Verification items for the finished model (mm, model axes). A direction names the side the tool comes from. Give positions to 0.01 mm unless a question says otherwise; leave off trailing zeros. Order: outer loops, then holes, each group sorted by start corner. A loop starts at its lowest first (then second) coordinate and runs counter-clockwise, first axis right, second up.
(1) Gauge pin test, flat ends, axial feed: pin 1 (1.2 mm diameter, centred on y = 44, z = 7.5, fed in from -X); pin 2 (4 mm diameter, centred on x = 20.17, y = 37.33, fed in from +Z); pin 3 (1.5 mm diameter, centred on x = 28, z = 3, fed in from -Y). Record the tip position at first contact, or that the pin passes through.
(2) Access from +Z, -Z, +X, -X, +Y, -Y to the whole of each face (thin tool, end or side, straight path). Record for faces 5 (the face through (21.836, 37.859, 6.084)), 6 (the face through (20.857, 39.996, 14.535)), 7 (the face through (10, 3, 7)).
(3) Sectioned sample at B-B on y = 20. Record the cut outline in (x, z).
(4) Mould release check, pull along X, two halves, no side actions. Record for faces 1 (the face through (42, 31, 8)), 2 (the face through (18, 32, 7)), 3 (the face through (33.794, 23.738, 14.535)), 4 (the face through (10, 60, 7)): pulls with the +X half, pulls with the -X half, needs draft (parallel to the pull), parting line crosses it, or undercut.
(5) Scan lines: L1, parallel to Y at x = 26, z = 9; L2, parallel to Z at x = 12, y = 17; L3, parallel to Y at x = 32, z = 14. Record each from-to range of solid material in increasing order.
(6) Sectioned sample at C-C on x = 26. Count the separate pieces of the cut face and the enclosed holes in it, plus the area to 3 significant figures.
(7) Sectioned sample at A-A on y = 31.5. Record the cut outline in (x, z), plus the area to 3 significant figures.
(8) Sectioned sample at D-D on y = 11.5. Record the cut outline in (x, z).
Autodesk Inventor part; units mm, degrees
ref_plane "Work Plane2" through (3, 0, 0) normal (-1, 0, 0) x (0, 0, 1)
ref_plane "YZ Plane" through (0, 0, 0) normal (1, 0, 0) x (0, 1, 0)
ref_plane "XZ Plane" through (0, 0, 0) normal (0, 1, 0) x (-1, 0, 0)
sketch "Sketch1" plane through (0, 0, 0) normal (0, 0, 1) x (1, 0, 0)
  line L0 (0, 0) -> (42, 0)
  line L1 (42, 0) -> (42, 63)
  line L2 (42, 63) -> (0, 63)
  line L3 (0, 63) -> (0, 0)
  dimension "d0" = 42
  dimension "d1" = 63
extrude "Extrusion1" add sketch "Sketch1" along normal blind 17
sketch "Sketch2" plane through (0, 0, 17) normal (0, 0, 1) x (1, 0, 0)
  line L0 (0, 63) -> (0, 0)
  line L1 (0, 31.5) -> (26, 31.5)
  circle A0 centre (26, 31.5) radius 5.25
  dimension "d4" = 26
  dimension "d5" = 10.5
extrude "Extrusion2" cut sketch "Sketch2" against normal blind 17
sketch "Sketch4" plane through (0, 0, 17) normal (0, 0, 1) x (1, 0, 0)
  circle A0 centre (26, 31.5) radius 5.25
  line L0 (26, 31.5) -> (26, 51.5)
  line L1 (26, 31.5) -> (26, 11.5)
  circle A1 centre (26, 51.5) radius 7.55
  circle A2 centre (26, 11.5) radius 7.55
  point P0 (0, 0)
  dimension "d14" = 20
  dimension "d15" = 20
  dimension "d16" = 15.1
  dimension "d17" = 15.1
extrude "Extrusion4" cut sketch "Sketch4" against normal blind 17 contours A2 | A1
sketch "Sketch5" plane through (0, 0, 17) normal (0, 0, 1) x (1, 0, 0)
  line L0 (0, 63) -> (0, 0)
  line L1 (0, 31.5) -> (10, 31.5)
  circle A0 centre (26, 31.5) radius 5.25
  line L2 (26, 31.5) -> (20.1664, 37.3336)
  line L3 (26, 31.5) -> (34.25, 31.5) construction
  line L4 (20.1664, 37.3336) -> (31.8336, 25.6664)
  circle A1 centre (31.8336, 25.6664) radius 1.75
  circle A2 centre (20.1664, 37.3336) radius 1.75
  dimension "d21" = 10
  dimension "d22" = 8.25
  dimension "d23" = 135
  dimension "d24" = 16.5
  dimension "d25" = 3.5
  dimension "d26" = 3.5
extrude "Extrusion5" cut sketch "Sketch5" against normal blind 17 contours A1 | A2
ref_plane "Work Plane1" through (0, 0, 7.5) normal (0, 0, 1) x (1, 0, 0)
sketch "Sketch8" plane through (0, 0, 17) normal (0, 0, 1) x (1, 0, 0)
  line L0 (0, 63) -> (0, 0)
  circle A0 centre (0, 31.5) radius 9.75
  dimension "d36" = 19.5
extrude "Extrusion8" cut sketch "Sketch8" against normal blind 10
sketch "Sketch9" plane through (0, 0, 7) normal (0, 0, 1) x (1, 0, 0)
  arc A0 (0, 21.75) -> (0, 41.25) centre (0, 31.5) ccw
  circle A1 centre (0, 31.5) radius 12.5
  point P0 (0, 0)
  dimension "d39" = 25
extrude "Extrusion9" [suppressed]
sketch "Sketch10" plane through (0, 0, 0) normal (-1, 0, 0) x (0, 0, 1)
  circle A0 centre (5, 6) radius 1.6
  line L0 (0, 26.25) -> (0, 36.75)
  line L1 (0, 31.5) -> (15.0441, 31.5)
  circle A1 centre (5, 57) radius 1.6
  point P0 (0, 0)
  dimension "d42" = 3.2
extrude "Extrusion10" [suppressed]
ref_plane "Work Plane2" through (3, 0, 0) normal (-1, 0, 0) x (0, 0, 1)
sketch "Sketch11" plane through (3, 0, 0) normal (-1, 0, 0) x (0, 0, 1)
  circle A0 centre (5, 6) radius 1.6
  line L0 (5, 6) -> (5, 8.75)
  line L1 (6.5877, 8.75) -> (8.1754, 6)
  line L2 (8.1754, 6) -> (6.5877, 3.25)
  line L3 (6.5877, 3.25) -> (3.4123, 3.25)
  line L4 (3.4123, 3.25) -> (1.8246, 6)
  line L5 (1.8246, 6) -> (3.4123, 8.75)
  line L6 (3.4123, 8.75) -> (6.5877, 8.75)
  circle A1 centre (5, 57) radius 1.6
  line L7 (5, 57) -> (5, 54.25)
  line L8 (3.4123, 54.25) -> (1.8246, 57)
  line L9 (1.8246, 57) -> (3.4123, 59.75)
  line L10 (3.4123, 59.75) -> (6.5877, 59.75)
  line L11 (6.5877, 59.75) -> (8.1754, 57)
  line L12 (8.1754, 57) -> (6.5877, 54.25)
  line L13 (6.5877, 54.25) -> (3.4123, 54.25)
  point P0 (0, 0)
  dimension "d46" = 2.75
  dimension "d47" = 2.75
extrude "Extrusion11" [suppressed]
sketch "Sketch12" plane through (0, 0, 0) normal (0, 0, -1) x (-1, 0, 0)
  line L0 (-3, 3.25) -> (-5.5, 3.25)
  line L1 (-3, 3.25) -> (-5.5, 3.25)
  line L2 (-5.5, 3.25) -> (-5.5, 8.75)
  line L3 (-5.5, 8.75) -> (-3, 8.75)
  line L4 (-3, 8.75) -> (-3, 3.25)
  line L5 (-3, 43.25) -> (-5.5, 43.25)
  line L6 (-5.5, 48.75) -> (-5.5, 46)
  line L7 (-3, 43.25) -> (-5.5, 43.25)
  line L8 (-5.5, 43.25) -> (-5.5, 48.75)
  line L9 (-5.5, 48.75) -> (-3, 48.75)
  line L10 (-3, 48.75) -> (-3, 43.25)
  point P0 (0, 0)
extrude "Extrusion12" [suppressed]
sketch "Sketch13" plane through (0, 0, 0) normal (-1, 0, 0) x (0, 0, 1)
  line L0 (5, 60) -> (9, 60)
  line L1 (9, 60) -> (9, 3)
  line L2 (9, 3) -> (5, 3)
  line L3 (5, 3) -> (5, 60)
  point P0 (0, 0)
  point P1 (5, 31.5)
  dimension "d83" = 4
extrude "Extrusion13" cut sketch "Sketch13" against normal blind 18
fillet "Fillet1" radius 2 2 edges at (0, 3, 7) (0, 60, 7)
sketch "Sketch14" plane through (0, 0, 0) normal (-1, 0, 0) x (0, 0, 1)
  point P0 (0, 0)
sketch "Sketch15" plane through (0, 0, 0) normal (0, 0, -1) x (-1, 0, 0)
  line L0 (0, 21.75) -> (0, 41.25)
  line L1 (0, 61.05) -> (0, 53.05)
  line L2 (0, 53.05) -> (-5, 53.05)
  circle A0 centre (-5, 53.05) radius 1.6
  line L3 (0, 0) -> (-42, 0)
  line L4 (0, 0) -> (0, 8)
  line L5 (-2, 11.95) -> (-10, 11.95)
  line L6 (0, 8) -> (-5, 8)
  circle A1 centre (-5, 8) radius 1.6
  point P0 (0, 9.95)
  dimension "d59" = 8
  dimension "d60" = 5
  dimension "d61" = 3.2
  dimension "d71" = 8
  dimension "d72" = 5
  dimension "d73" = 3.2
extrude "Extrusion14" [suppressed]
sketch "Sketch17" plane through (0, 0, 17) normal (0, 0, 1) x (1, 0, 0)
  circle A0 centre (5, 53.05) radius 1.6
  line L0 (5, 53.05) -> (5, 50.3)
  line L1 (3.4123, 50.3) -> (1.8246, 53.05)
  line L2 (1.8246, 53.05) -> (3.4123, 55.8)
  line L3 (3.4123, 55.8) -> (6.5877, 55.8)
  line L4 (6.5877, 55.8) -> (8.1754, 53.05)
  line L5 (8.1754, 53.05) -> (6.5877, 50.3)
  line L6 (6.5877, 50.3) -> (3.4123, 50.3)
  circle A1 centre (5, 8) radius 1.6
  line L7 (5, 8) -> (5, 10.75)
  line L8 (6.5877, 10.75) -> (8.1754, 8)
  line L9 (8.1754, 8) -> (6.5877, 5.25)
  line L10 (6.5877, 5.25) -> (3.4123, 5.25)
  line L11 (3.4123, 5.25) -> (1.8246, 8)
  line L12 (1.8246, 8) -> (3.4123, 10.75)
  line L13 (3.4123, 10.75) -> (6.5877, 10.75)
  point P0 (0, 0)
  dimension "d68" = 2.75
  dimension "d76" = 2.75
extrude "Extrusion15" [suppressed]
sketch "Sketch19" plane through (0, 0, 0) normal (-1, 0, 0) x (0, 0, 1)
  point P0 (0, 0)
sketch "Sketch20" plane through (0, 0, 0) normal (-1, 0, 0) x (0, 0, 1)
  point P0 (0, 0)
fillet "Fillet2" radius 4 4 edges at (21, 0, 0) (21, 63, 0) (21, 63, 17) (21, 0, 17)
sketch "Sketch21" plane through (0, 0, 17) normal (0, 0, 1) x (1, 0, 0)
  circle A0 centre (31.8336, 25.6664) radius 1.75
  line L0 (31.8336, 25.6664) -> (29.8891, 27.6109)
  line L1 (31.8336, 25.6664) -> (34.5836, 25.6664) construction
  circle A1 centre (20.1664, 37.3336) radius 1.75
  line L2 (20.1664, 37.3336) -> (22.1109, 35.3891)
  line L3 (20.9882, 34.2664) -> (17.921, 35.0883)
  line L4 (17.921, 35.0883) -> (17.0991, 38.1555)
  line L5 (17.0991, 38.1555) -> (19.3445, 40.4009)
  line L6 (19.3445, 40.4009) -> (22.4117, 39.579)
  line L7 (22.4117, 39.579) -> (23.2336, 36.5118)
  line L8 (23.2336, 36.5118) -> (20.9882, 34.2664)
  line L9 (31.0118, 28.7336) -> (34.079, 27.9117)
  line L10 (34.079, 27.9117) -> (34.9009, 24.8445)
  line L11 (34.9009, 24.8445) -> (32.6555, 22.5991)
  line L12 (32.6555, 22.5991) -> (29.5883, 23.421)
  line L13 (29.5883, 23.421) -> (28.7664, 26.4882)
  line L14 (28.7664, 26.4882) -> (31.0118, 28.7336)
  point P0 (0, 0)
  dimension "d78" = 2.75
  dimension "d79" = 135
  dimension "d80" = 2.75
extrude "Extrusion16" cut sketch "Sketch21" against normal blind 5
chamfer "Chamfer1" distance 2.5 angle 45 8 edges at (42, 31.5, 17) (42, 61.8284, 15.8284) (42, 63, 8.5) (42, 61.8284, 1.1716) (42, 31.5, 0) (42, 1.1716, 1.1716) (42, 0, 8.5) (42, 1.1716, 15.8284)
properties part number "syringe_pump_sledge"
Ans:
1. pin 1: stops at x = 18
1. pin 2: stops at z = 12
1. pin 3: stops at y = 0.01
2. face 5: +Z, -Z
2. face 6: +Z
2. face 7: -X
3. outline: (0, 0) - (39.5, 0) - (42, 2.5) - (42, 14.5) - (39.5, 17) - (0, 17) - (0, 9) - (18, 9) - (18, 5) - (0, 5) - close
4. face 1: pulls with the +X half
4. face 2: pulls with the -X half
4. face 3: undercut
4. face 4: needs draft
5. L1: y = 0 to 3.95, 19.05 to 26.25, 36.75 to 43.95, 59.05 to 63
5. L2: z = 0 to 5, 9 to 17
5. L3: y = 0.13 to 6.92, 16.08 to 22.77, 28.47 to 46.92, 56.08 to 62.87
6. separate pieces: 4
6. enclosed holes: 0
6. area: 365 mm2
7. outline: (0, 0) - (20.75, 0) - (20.75, 17) - (9.75, 17) - (9.75, 9) - (18, 9) - (18, 5) - (0, 5) - close; (31.25, 0) - (39.5, 0) - (42, 2.5) - (42, 14.5) - (39.5, 17) - (31.25, 17) - close
7. area: 379 mm2
8. outline: (0, 0) - (18.45, 0) - (18.45, 17) - (0, 17) - (0, 9) - (18, 9) - (18, 5) - (0, 5) - close; (33.55, 0) - (39.5, 0) - (42, 2.5) - (42, 14.5) - (39.5, 17) - (33.55, 17) - close
